```python
from build123d import *

# Parameters (mm, degrees)
SKETCH1_W           = 43
SKETCH1_H           = 18
BOSS_EXTRUDE1_DEPTH = 8
CAVITY2_DEPTH       = 2.3
BOSS_EXTRUDE2_DEPTH = 4


# Read off the part's stored shape, not the designer's step: Cavity2
with BuildPart() as part:
    # Sketch1 → Boss-Extrude1 (new body)
    with BuildSketch(Plane.XY):
        Rectangle(SKETCH1_W, SKETCH1_H)
    extrude(amount=BOSS_EXTRUDE1_DEPTH)

    # Cavity2 outline → Cavity2 (cut)
    with BuildSketch(Plane.XY):
        with BuildLine():
            ThreePointArc((-4.514897629, -4.536044466), (0, -6.4), (4.514897629, -4.536044466))
            Line((4.514897629, -4.536044466), (17, -2.7))
            ThreePointArc((17, -2.7), (19.7, 0), (17, 2.7))
            Line((17, 2.7), (4.514897629, 4.536044466))
            ThreePointArc((4.514897629, 4.536044466), (0, 6.4), (-4.514897629, 4.536044466))
            Line((-4.514897629, 4.536044466), (-17, 2.7))
            ThreePointArc((-17, 2.7), (-19.7, 0), (-17, -2.7))
            Line((-17, -2.7), (-4.514897629, -4.536044466))
        make_face()
    extrude(amount=CAVITY2_DEPTH, mode=Mode.SUBTRACT)

    # Sketch4 → Boss-Extrude2 (add)
    with BuildSketch(Plane.XY.offset(8)):
        with BuildLine():
            ThreePointArc((-56.5, 0), (-57.964466094, 3.535533906), (-61.5, 5))
            Line((-61.5, 5), (-61.5, 2))
            ThreePointArc((-61.5, 2), (-60.085786438, 1.414213562), (-59.5, 0))
            ThreePointArc((-59.5, 0), (-60.085786438, -1.414213562), (-61.5, -2))
            Line((-61.5, -2), (-61.5, -5))
            ThreePointArc((-61.5, -5), (-57.964466094, -3.535533906), (-56.5, 0))
        make_face()
        with BuildLine():
            Line((-61.5, 2), (-61.5, 5))
            ThreePointArc((-61.5, 5), (-66.5, 0), (-61.5, -5))
            Line((-61.5, -5), (-61.5, -2))
            ThreePointArc((-61.5, -2), (-63.5, 0), (-61.5, 2))
        make_face()
        with BuildLine():
            Line((-21.5, -5), (-21.5, 5))
            Line((-21.5, 5), (-61.5, 5))
            ThreePointArc((-61.5, 5), (-57.964466094, 3.535533906), (-56.5, 0))
            ThreePointArc((-56.5, 0), (-57.964466094, -3.535533906), (-61.5, -5))
            Line((-61.5, -5), (-21.5, -5))
        make_face()
    extrude(amount=-BOSS_EXTRUDE2_DEPTH)


solid = part.part
```
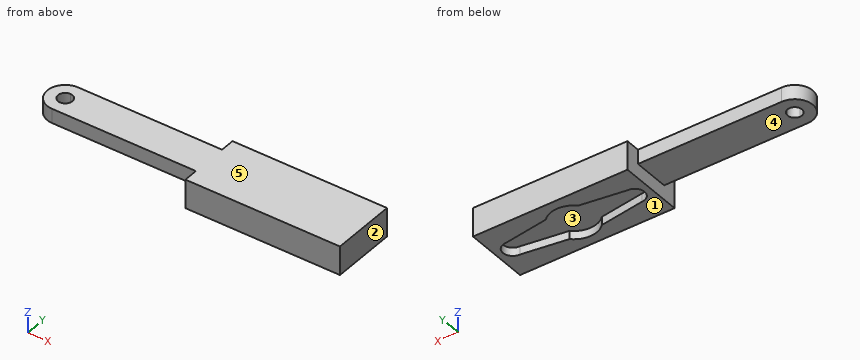
Verification items for the finished model (mm, model axes). Face numbers are marked on the shaded views. A direction names the side the tool comes from. Give positions to 0.01 mm unless a question says otherwise; leave off trailing zeros. Order: outer loops, then holes, each group sorted by start corner. A loop starts at its lowest first (then second) coordinate and runs counter-clockwise, first axis right, second up. Notation, with made-up numbers: (25.25, 5.25) -> (44.25, 5.25) arc R37 cw to (44.25, 42.25) -> close; hole circle Ø2 at (59.5, 18.5). An arc over 180 degrees is marked (long way). Use a Markdown table: item, result.
1) Section check D-D, the plane x = -54.5. Record the boundary of the cut face in (y, z), then the cut area to 3 significant figures.
Results:
| item | result |
|---|---|
| outline | (-5, 4) -> (5, 4) -> (5, 8) -> (-5, 8) -> close |
| area | 40.0 mm² |
2) Section check C-C, the plane z = 3.25. Record the boundary of the cut face in (x, y).
Results:
| item | result |
|---|---|
| outline | (-21.5, -9) -> (21.5, -9) -> (21.5, 9) -> (-21.5, 9) -> close |
3) Mould release check, pull along X, two halves, no side actions. Record for the marked faces 1, 2 and 3: pulls with the +X half, pulls with the -X half, needs draft (parallel to the pull), parting line crosses it, or undercut.
Results:
| item | result |
|---|---|
| face 1 | needs draft |
| face 2 | pulls with the +X half |
| face 3 | undercut |
4) Material ranges on probe 1 along Z at (x, y) = (-10.5, -1); probe 2 along Y at (x, z) = (12, 2); probe 3 along Z at (x, y) = (-56, 4.25), recorded low to high.
Results:
| item | result |
|---|---|
| probe 1 | 2.3 to 8 |
| probe 2 | -9 to -3.44, 3.44 to 9 |
| probe 3 | 4 to 8 |
5) Section check B-B, the plane y = -3.75. Record the boundary of the cut face in (x, z).
Results:
| item | result |
|---|---|
| outline | (-64.81, 4) -> (-21.5, 4) -> (-21.5, 0) -> (-9.86, 0) -> (-9.86, 2.3) -> (9.86, 2.3) -> (9.86, 0) -> (21.5, 0) -> (21.5, 8) -> (-64.81, 8) -> close |
6) Section check A-A, the plane x = 7.5. Record the boundary of the cut face in (y, z).
Results:
| item | result |
|---|---|
| outline | (-9, 0) -> (-4.1, 0) -> (-4.1, 2.3) -> (4.1, 2.3) -> (4.1, 0) -> (9, 0) -> (9, 8) -> (-9, 8) -> close |
7) Tool access check on the marked faces 4 and 5. Record the directions out of +Z, -Z, +X, -X, +Y, -Y that give a thin tool (end or side, any length) a straight path to the whole face; none if there is none.
Results:
| item | result |
|---|---|
| face 4 | -Z, -X, +Y, -Y |
| face 5 | +Z, +X, -X, +Y, -Y |
8) Depth check by flat-ended pin: pin 1 Ø2 at (y, z) = (-2.5, 2.5) entering from -X; pin 2 Ø4.5 at (x, z) = (-46, 5.5) entering from -Y; pin 3 Ø2 at (x, y) = (-54, 0) entering from -Z. Enter the tip coordinate at first touch or a pass-through.
Results:
| item | result |
|---|---|
| pin 1 | x = -21.5 |
| pin 2 | y = -5 |
| pin 3 | z = 4 |
